Design review of the part built by this model. Coordinates are the model's own, in mm. A direction names the side the tool comes from. Coordinates: 2 decimals unless noted, no trailing zeros. Write each loop counter-clockwise with the first axis right and the second up, starting at its lowest first coordinate (ties: lowest second). Pieces come first, ordered by that corner, then holes. Notation, with made-up numbers: (28, -18) -> (54, -18) arc R20 ccw to (54, 6) -> close; hole circle Ø11 at (80, 87). An arc over 180 degrees is marked (long way). Answer in a Markdown table with one row per item. Add a question column.
Item 1: Take a section at D-D, the plane y = 6. Write out the cut boundary in (x, z), and give its area (3 significant figures).
Item 2: Take a section at C-C, the plane z = 52. Write out the cut boundary in (x, y), and give its area (3 significant figures).
Item 3: Take a section at A-A, the plane y = 16. Write out the cut boundary in (x, z) (3 decimals), and give its area (3 significant figures).
Item 4: Draft analysis for pull direction Y (two halves, no side actions). For faces 1 (the face through (19, -14, 31)), 2 (the face through (2, 7.2, 13.6)), 3 (the face through (0, 6, 32)), state which applies: released by +Y, released by -Y, zero draft, split by the parting line, or undercut.
Item 5: Clearance check with flat-ended pins moving along their axes: P1, Ø3.5, axis at y = 6, z = 12, coming from the -X side; P2, Ø3.5, axis at y = 8, z = 18, coming from the +X side; P3, Ø2, axis at x = 29, y = -9.5, coming from the +Z side; P4, Ø6, axis at x = 15.5, y = 11, coming from the +Z side. State where each tip first meets the part, or that it passes through.
Item 6: Take a section at B-B, the plane x = 3. Write out the cut boundary in (y, z).
Item 7: To check wall thickness, follow line 1 (Z direction, x = 1.5, y = 6); line 2 (Y direction, x = 2, z = 20); line 3 (X direction, y = 10, z = 10.5). State the ranges of each line that lie inside material, in increasing order.
Item 8: For faces 4 (the face through (7, 6, 38.5)), 5 (the face through (4, -7, 32)), 6 (the face through (19, 6, 32)), list the 3-axis set-ups (+Z, -Z, +X, -X, +Y, -Y) from which the entire face can be reached by the end or side of a thin tool; tool diameter is ignored.
Autodesk Fusion 360 part; units mm, degrees
sketch "Sketch1" plane through (0, 0, 0) normal (0, 0, 1) x (1, 0, 0)
  line L0 (0, 0) -> (4, 0)
  line L1 (4, 0) -> (4, 12)
  line L2 (4, 12) -> (0, 12)
  line L3 (0, 12) -> (0, 0)
  dimension "d1" = 12
  dimension "d2" = 4
extrude "Extrude1" add sketch "Sketch1" along normal blind 64
sketch "Sketch2" plane through (4, 0, 0) normal (1, 0, 0) x (0, 1, 0)
  line L0 (0, 0) -> (12, 0)
  line L1 (12, 0) -> (12, 64)
  line L2 (12, 64) -> (0, 64)
  line L3 (0, 64) -> (0, 0)
  line L4 (0, 64) -> (12, 0) construction
  line L5 (12, 64) -> (0, 0) construction
  line L6 (12, 38.5) -> (0, 38.5)
  line L7 (0, 38.5) -> (0, 25.5)
  line L8 (0, 25.5) -> (12, 25.5)
  line L9 (12, 25.5) -> (12, 38.5)
  line L10 (12, 38.5) -> (0, 25.5) construction
  line L11 (0, 38.5) -> (12, 25.5) construction
  line L12 (6, 32) -> (6, 36) construction
  line L13 (6, 36) -> (6, 44) construction
  line L14 (6, 44) -> (6, 52) construction
  line L15 (6, 32) -> (6, 28) construction
  line L16 (6, 28) -> (6, 20) construction
  line L17 (6, 20) -> (6, 12) construction
  point P0 (6, 32)
  point P1 (6, 52)
  point P2 (6, 44)
  point P3 (6, 36)
  point P4 (6, 28)
  point P5 (6, 20)
  point P6 (6, 12)
  dimension "d5" = 13
  dimension "d6" = 4
  dimension "d7" = 8
  dimension "d8" = 8
  dimension "d9" = 4
  dimension "d10" = 8
  dimension "d11" = 8
  dimension "d20" = 12
extrude "Extrude2" add sketch "Sketch2" along normal blind 5 contours L1 L3 L6 L7 L8 L9
sketch "Sketch3" plane through (9, 0, 0) normal (1, 0, 0) x (0, 1, 0)
  line L0 (12, 25.5) -> (12, 38.5)
  line L1 (12, 38.5) -> (0, 38.5)
  line L2 (0, 38.5) -> (0, 25.5)
  line L3 (0, 25.5) -> (12, 25.5)
  line L4 (0, 25.5) -> (12, 25.5)
  line L5 (12, 25.5) -> (12, 32)
  line L6 (12, 32) -> (0, 32)
  line L7 (0, 32) -> (0, 25.5)
extrude "Extrude3" add sketch "Sketch3" along normal blind 20.11 contours L0 L2 L3 L4 L5 L6 L7
sketch "Sketch4" plane through (29.11, 0, 0) normal (1, 0, 0) x (0, 1, 0)
  line L0 (0, 32) -> (0, 25.5)
  line L1 (0, 25.5) -> (12, 25.5)
  line L2 (12, 25.5) -> (12, 32)
  line L3 (12, 32) -> (0, 32)
  line L4 (0, 25.5) -> (12, 25.5)
  line L5 (12, 25.5) -> (12, 38.5)
  line L6 (12, 38.5) -> (0, 38.5)
  line L7 (0, 38.5) -> (0, 25.5)
  dimension "d16" = 12
  dimension "d17" = 13
extrude "Extrude4" add sketch "Sketch4" along normal blind 5
sketch "Sketch5" plane through (0, 0, 32) normal (0, 0, 1) x (-1, 0, 0)
  line L0 (-9, -12) -> (-9, 0)
  line L1 (-9, 0) -> (-29.11, 0)
  line L2 (-29.11, 0) -> (-29.11, -12)
  line L3 (-29.11, -12) -> (-9, -12)
hole "Hole1" at (4, 6, 52) at (4, 6, 44) at (4, 6, 20) at (4, 6, 12) direction (-1, 0, 0) diameter 4 depth 15 tip angle 180
sketch "Sketch6" plane through (0, 12, 0) normal (0, 1, 0) x (-1, 0, 0)
  line L0 (-4, 0) -> (0, 0)
  line L1 (0, 0) -> (0, 64)
  line L2 (0, 64) -> (-4, 64)
  line L3 (-4, 64) -> (-4, 38.5)
  line L4 (-4, 38.5) -> (-9, 38.5)
  line L5 (-9, 38.5) -> (-9, 32)
  line L6 (-9, 32) -> (-29.11, 32)
  line L7 (-29.11, 32) -> (-29.11, 38.5)
  line L8 (-29.11, 38.5) -> (-34.11, 38.5)
  line L9 (-34.11, 38.5) -> (-34.11, 25.5)
  line L10 (-34.11, 25.5) -> (-4, 25.5)
  line L11 (-4, 25.5) -> (-4, 0)
  line L12 (-4, 38.5) -> (-4, 25.5)
  line L13 (-4, 38.5) -> (-9, 38.5)
  line L14 (-9, 38.5) -> (-9, 32)
  line L15 (-9, 32) -> (-29.11, 32)
  line L16 (-29.11, 38.5) -> (-29.11, 32)
  line L17 (-29.11, 38.5) -> (-34.11, 38.5)
  line L18 (-34.11, 25.5) -> (-34.11, 38.5)
  line L19 (-4, 25.5) -> (-34.11, 25.5)
extrude "Extrude5" add sketch "Sketch6" along normal blind 14 contours L4 L5 L6 L7 L8 L9 L10 L12 L13 L14 L15 L16 L17 L18 L19
sketch "Sketch7" plane through (0, 0, 0) normal (0, -1, 0) x (1, 0, 0)
  line L0 (0, 0) -> (4, 0)
  line L1 (4, 0) -> (4, 25.5)
  line L2 (4, 25.5) -> (34.11, 25.5)
  line L3 (34.11, 25.5) -> (34.11, 38.5)
  line L4 (34.11, 38.5) -> (29.11, 38.5)
  line L5 (29.11, 38.5) -> (29.11, 32)
  line L6 (29.11, 32) -> (9, 32)
  line L7 (9, 32) -> (9, 38.5)
  line L8 (9, 38.5) -> (4, 38.5)
  line L9 (4, 38.5) -> (4, 64)
  line L10 (4, 64) -> (0, 64)
  line L11 (0, 64) -> (0, 0)
  line L12 (4, 38.5) -> (4, 25.5)
  line L13 (4, 25.5) -> (34.11, 25.5)
  line L14 (34.11, 25.5) -> (34.11, 38.5)
  line L15 (34.11, 38.5) -> (29.11, 38.5)
  line L16 (29.11, 38.5) -> (29.11, 32)
  line L17 (29.11, 32) -> (9, 32)
  line L18 (9, 32) -> (9, 38.5)
  line L19 (9, 38.5) -> (4, 38.5)
extrude "Extrude6" add sketch "Sketch7" along normal blind 14 contours L2 L3 L4 L5 L6 L7 L8 L12 L13 L14 L15 L16 L17 L18 L19
sketch "Sketch8" plane through (0, 0, 32) normal (0, 0, 1) x (-1, 0, 0)
  line L0 (-9, -26) -> (-9, 14)
  line L1 (-9, 14) -> (-29.11, 14)
  line L2 (-29.11, 14) -> (-29.11, -26)
  line L3 (-29.11, -26) -> (-9, -26)
  line L4 (-9, -26) -> (-29.11, 14) construction
  line L5 (-29.11, -26) -> (-9, 14) construction
  line L6 (-19.055, -6) -> (-19.055, -16) construction
  line L7 (-19.055, -6) -> (-19.055, 4)
  dimension "d28" = 10
  dimension "d29" = 10
hole "Hole2" at (19.055, -4, 32) at (19.055, 16, 32) direction (0, 0, -1) diameter 4 depth 50 tip angle 180
Answers:
| question | item | result |
|---|---|---|
| 1 | outline | (0, 0) -> (4, 0) -> (4, 10) -> (0, 10) -> close; (0, 14) -> (4, 14) -> (4, 18) -> (0, 18) -> close; (0, 22) -> (4, 22) -> (4, 25.5) -> (34.11, 25.5) -> (34.11, 38.5) -> (29.11, 38.5) -> (29.11, 32) -> (9, 32) -> (9, 38.5) -> (4, 38.5) -> (4, 42) -> (0, 42) -> close; (0, 46) -> (4, 46) -> (4, 50) -> (0, 50) -> close; (0, 54) -> (4, 54) -> (4, 64) -> (0, 64) -> close |
| 1 | area | 453 mm^2 |
| 2 | outline | (0, 0) -> (4, 0) -> (4, 4) -> (0, 4) -> close; (0, 8) -> (4, 8) -> (4, 12) -> (0, 12) -> close |
| 2 | area | 32.0 mm^2 |
| 3 | outline | (4, 25.5) -> (17.055, 25.5) -> (17.055, 32) -> (9, 32) -> (9, 38.5) -> (4, 38.5) -> close; (21.055, 25.5) -> (34.11, 25.5) -> (34.11, 38.5) -> (29.11, 38.5) -> (29.11, 32) -> (21.055, 32) -> close |
| 3 | area | 235 mm^2 |
| 4 | face 1 | released by -Y |
| 4 | face 2 | undercut |
| 4 | face 3 | zero draft |
| 5 | P1 | passes through |
| 5 | P2 | stops at x = 4 |
| 5 | P3 | stops at z = 38.5 |
| 5 | P4 | stops at z = 32 |
| 6 | outline | (0, 0) -> (12, 0) -> (12, 64) -> (0, 64) -> close; hole circle Ø4 at (6, 12); hole circle Ø4 at (6, 20); hole circle Ø4 at (6, 44); hole circle Ø4 at (6, 52) |
| 7 | line 1 | z = 0 to 10, 14 to 18, 22 to 42, 46 to 50, 54 to 64 |
| 7 | line 2 | y = 0 to 4, 8 to 12 |
| 7 | line 3 | x = 0 to 4 |
| 8 | face 4 | +Z, +X, +Y, -Y |
| 8 | face 5 | +Z, -Z, -X, -Y |
| 8 | face 6 | +Z, +Y, -Y |
